Geometry check sheet. Reference: the model listing, model coordinates, mm. Coordinates: 2 decimals unless noted, no trailing zeros. One line per item, written item: value.
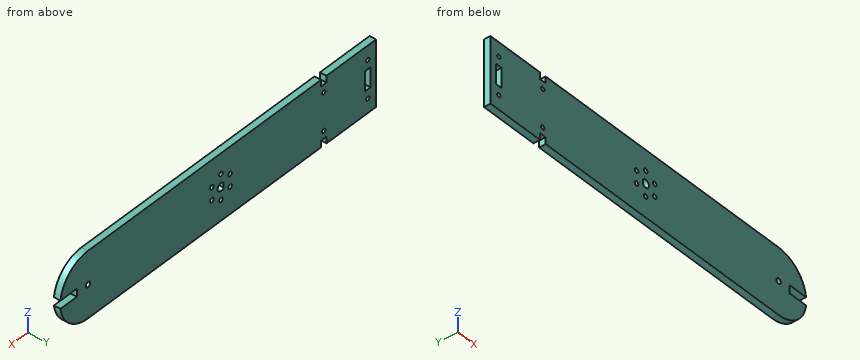
from build123d import *

# Parameters (mm, degrees)
CROQUIS1_R              = 1.5
CROQUIS1_R_2            = 1.63
CROQUIS1_R_3            = 2
CROQUIS1_W              = 5
CROQUIS1_H              = 15
SALIENTE_EXTRUIR1_DEPTH = 5


with BuildPart() as part:
    # Croquis1 → Saliente-Extruir1 (new body)
    with BuildSketch(Plane(origin=(0, 0, 0), x_dir=(1, 0, 0), z_dir=(0, 1, 0))):
        with BuildLine():
            Line((0, 0), (44.75, 0))
            Line((44.75, 0), (44.75, 5))
            Line((44.75, 5), (49.75, 5))
            Line((49.75, 5), (49.75, 0))
            Line((49.75, 0), (260, 0))
            ThreePointArc((260, 0), (276.583123952, 6.291713066), (284.819347292, 22))
            Line((284.819347292, 22), (270, 22))
            Line((270, 22), (270, 28))
            Line((270, 28), (284.819347292, 28))
            ThreePointArc((284.819347292, 28), (276.583123952, 43.708286934), (260, 50))
            Line((260, 50), (49.75, 50))
            Line((49.75, 50), (49.75, 45))
            Line((49.75, 45), (44.75, 45))
            Line((44.75, 45), (44.75, 50))
            Line((44.75, 50), (0, 50))
            Line((0, 50), (0, 0))
        make_face()
        with Locations(Location((47.25, 39.25, 0), (0, 0, 270))):
            Circle(CROQUIS1_R, mode=Mode.SUBTRACT)
        with Locations(Location((140, 34.5, 0), (0, 0, 270))):
            Circle(CROQUIS1_R_2, mode=Mode.SUBTRACT)
        with Locations(Location((47.25, 10.75, 0), (0, 0, 90))):
            Circle(CROQUIS1_R, mode=Mode.SUBTRACT)
        with Locations(Location((7.5, 10.75, 0), (0, 0, 270))):
            Circle(CROQUIS1_R, mode=Mode.SUBTRACT)
        with Locations(Location((7.5, 39.25, 0), (0, 0, 90))):
            Circle(CROQUIS1_R, mode=Mode.SUBTRACT)
        with Locations(Location((131.772758664, 29.75, 0), (0, 0, 270))):
            Circle(CROQUIS1_R_2, mode=Mode.SUBTRACT)
        with Locations(Location((131.772758664, 20.25, 0), (0, 0, 270))):
            Circle(CROQUIS1_R_2, mode=Mode.SUBTRACT)
        with Locations(Location((140, 15.5, 0), (0, 0, 270))):
            Circle(CROQUIS1_R_2, mode=Mode.SUBTRACT)
        with Locations(Location((148.227241336, 20.25, 0), (0, 0, 270))):
            Circle(CROQUIS1_R_2, mode=Mode.SUBTRACT)
        with Locations(Location((148.227241336, 29.75, 0), (0, 0, 270))):
            Circle(CROQUIS1_R_2, mode=Mode.SUBTRACT)
        with Locations(Location((260, 25, 0), (0, 0, 270))):
            Circle(CROQUIS1_R_3, mode=Mode.SUBTRACT)
        with Locations((7.5, 25)):
            Rectangle(CROQUIS1_W, CROQUIS1_H, mode=Mode.SUBTRACT)
        with BuildLine():
            Line((137.6, 23.2), (137.6, 26.8))
            ThreePointArc((137.6, 26.8), (143, 25), (137.6, 23.2))
        make_face(mode=Mode.SUBTRACT)
    extrude(amount=SALIENTE_EXTRUIR1_DEPTH)


solid = part.part
(1) Material ranges on probe 1 along Z at (x, y) = (260, 2.7); probe 2 along Z at (x, y) = (133, 2.8); probe 3 along X at (y, z) = (1.85, -26.5), recorded low to high. Write a range as from..to.
Reply:
probe 1: -50..-27, -23..0
probe 2: -50..-30.82, -28.68..-21.32, -19.18..0
probe 3: 0..5, 10..137.6, 142.6..258.68, 261.32..270
(2) Go/stop test with flat-tipped pins: pin 1 Ø1 at (y, z) = (1.5, -20) entering from +X; pin 2 Ø1.5 at (x, y) = (46, 2.5) entering from +Z; pin 3 Ø1.8 at (y, z) = (2, -24.5) entering from +X. Record where each tip stops, or that it passes through.
Reply:
pin 1: x = 284.59
pin 2: z = -5
pin 3: x = 270
(3) Cross-section at A-A on y = 2.25. State how many separate pieces and enclosed holes the cut face has, and give its area (3 significant figures).
Reply:
separate pieces: 1
enclosed holes: 13
area: 13,600 mm2
